Autodesk Inventor part; units mm, degrees
ref_plane "YZ Plane" through (0, 0, 0) normal (1, 0, 0) x (0, 1, 0)
ref_plane "XZ Plane" through (0, 0, 0) normal (0, 1, 0) x (-1, 0, 0)
ref_plane "XY Plane" through (0, 0, 0) normal (0, 0, 1) x (1, 0, 0)
sketch "Sketch1" plane through (0, 0, 0) normal (0, 0, 1) x (1, 0, 0)
  line L0 (0, 0) -> (-203.2, 0)
  line L1 (-203.2, 0) -> (-203.2, -1.6002)
  line L2 (-203.2, -1.6002) -> (0, -1.6002)
  line L3 (0, -1.6002) -> (0, 0)
  dimension "d0" = 203.2
  dimension "d1" = 1.6002
extrude "Extrusion1" add sketch "Sketch1" along normal blind 86.36
sketch "Sketch2" plane through (-203.2, 0, 0) normal (0, 1, 0) x (1, 0, 0)
  line L0 (203.2, 0) -> (0, 0)
  line L1 (203.2, -86.36) -> (0, -86.36)
  line L2 (0, 0) -> (1.6002, 0)
  line L3 (1.6002, 0) -> (1.6002, -86.36)
  line L4 (1.6002, -86.36) -> (0, -86.36)
  line L5 (0, -86.36) -> (0, 0)
  dimension "d4" = 1.6002
extrude "Extrusion2" add sketch "Sketch2" along normal blind 15.24
sketch "Sketch3" plane through (0, 0, 86.36) normal (0, 1, 0) x (1, 0, 0)
  line L0 (-203.2, 0) -> (0, 0)
  line L1 (-203.2, 86.36) -> (0, 86.36)
  line L2 (-150.7998, 0) -> (-149.1996, 0)
  line L3 (-149.1996, 0) -> (-149.1996, 86.36)
  line L4 (-149.1996, 86.36) -> (-150.7998, 86.36)
  line L5 (-150.7998, 86.36) -> (-150.7998, 0)
  dimension "d7" = 1.6002
extrude "Extrusion3" add sketch "Sketch3" along normal blind 15.24
sketch "Sketch4" plane through (0, 0, 86.36) normal (0, 1, 0) x (1, 0, 0)
  line L0 (-203.2, 0) -> (0, 0)
  line L1 (-203.2, 86.36) -> (0, 86.36)
  line L2 (-98.3996, 0) -> (-96.7994, 0)
  line L3 (-96.7994, 0) -> (-96.7994, 86.36)
  line L4 (-96.7994, 86.36) -> (-98.3996, 86.36)
  line L5 (-98.3996, 86.36) -> (-98.3996, 0)
  dimension "d10" = 1.6002
extrude "Extrusion4" add sketch "Sketch4" along normal blind 15.24
sketch "Sketch5" plane through (0, 0, 86.36) normal (0, 1, 0) x (1, 0, 0)
  line L0 (0, 0) -> (-96.7994, 0)
  line L1 (0, 86.36) -> (-96.7994, 86.36)
  line L2 (-45.9994, 0) -> (-44.3992, 0)
  line L3 (-44.3992, 0) -> (-44.3992, 86.36)
  line L4 (-44.3992, 86.36) -> (-45.9994, 86.36)
  line L5 (-45.9994, 86.36) -> (-45.9994, 0)
  dimension "d13" = 1.6002
extrude "Extrusion5" add sketch "Sketch5" along normal blind 15.24
sketch "Sketch6" plane through (-203.2, -1.6002, 0) normal (-1, 0, 0) x (0, 0, 1)
  line L0 (0, 0) -> (86.36, 0)
  line L1 (36.83, 0) -> (49.53, 0)
  line L2 (49.53, 0) -> (49.53, 80.01)
  line L3 (49.53, 80.01) -> (36.83, 80.01)
  line L4 (36.83, 80.01) -> (36.83, 0)
  point P0 (0, 1.6002)
  dimension "d16" = 12.7
  dimension "d17" = 80.01
extrude "Extrusion6" add sketch "Sketch6" along normal blind 1.6002
sketch "Sketch7" plane through (0, 0, 86.36) normal (1, 0, 0) x (0, 0, -1)
  line L0 (36.83, -1.6002) -> (0, -1.6002)
  line L1 (49.53, 78.4098) -> (49.53, -1.6002)
  line L2 (36.83, -1.6002) -> (49.53, -1.6002)
  line L3 (49.53, -1.6002) -> (49.53, 78.4098)
  line L4 (49.53, 78.4098) -> (36.83, 78.4098)
  line L5 (36.83, 78.4098) -> (36.83, -1.6002)
  point P0 (86.36, 0)
  dimension "d20" = 80.01
extrude "Extrusion7" add sketch "Sketch7" along normal blind 1.6002
sketch "Sketch8" plane through (-96.7994, 0, 86.36) normal (0, 1, 0) x (1, 0, 0)
  point P0 (96.7994, 86.36)
properties part number "ModulePlate2.0"
Can you work these out from the model? Positions are in its coordinate system, mm. A direction names the side the tool comes from. Give positions to 0.01 mm unless a question says otherwise; leave off trailing zeros. Order: outer loops, then holes, each group sorted by start corner. A loop starts at its lowest first (then second) coordinate and runs counter-clockwise, first axis right, second up. Notation, with made-up numbers: M -11,20 L 27,20 A26 cw 27,49 Z; hole C 1.5,-27.75 d3. An arc over 180 degrees is marked long. One line per item, written item: value.
Item 1: If we section it at C-C on x = -59: Write out the boundary of the cut face in (y, z), and give its area (3 significant figures).
Verdict:
outline: M -1.6,0 L 0,0 L 0,86.36 L -1.6,86.36 Z
area: 138 mm2
Item 2: If we section it at A-A on y = 49: Write out the boundary of the cut face in (x, z).
Verdict:
outline: M -204.8,36.83 L -203.2,36.83 L -203.2,49.53 L -204.8,49.53 Z; M 0,36.83 L 1.6,36.83 L 1.6,49.53 L 0,49.53 Z
Item 3: For faces 4 (the face through (-203.2, 7, 68)), 5 (the face through (-149.2, 8, 44)), 6 (the face through (-102, -1, 86.36)), which set-ups out of +Z, -Z, +X, -X, +Y, -Y let a thin tool reach every point of the face, with its end or its side?
Verdict:
face 4: +Z, -X, +Y, -Y
face 5: +Z, -Z, +Y
face 6: +Z, +X, -X, +Y, -Y
Item 4: If we section it at B-B on z = 56: Write out the boundary of the cut face in (x, y), and give its area (3 significant figures).
Verdict:
outline: M -203.2,-1.6 L 0,-1.6 L 0,0 L -44.4,0 L -44.4,15.24 L -46,15.24 L -46,0 L -96.8,0 L -96.8,15.24 L -98.4,15.24 L -98.4,0 L -149.2,0 L -149.2,15.24 L -150.8,15.24 L -150.8,0 L -201.6,0 L -201.6,15.24 L -203.2,15.24 Z
area: 423 mm2
Item 5: If we mould it in two halves opening along X, with no side actions, what happens to faces 1 (the face through (-150.8, 8, 43)), 2 (the face through (-204.8, 39, 43)), 3 (the face through (-103, -1.6, 44))? For each: pulls with the +X half, pulls with the -X half, needs draft (parallel to the pull), parting line crosses it, or undercut.
Verdict:
face 1: undercut
face 2: pulls with the -X half
face 3: needs draft
Item 6: Please list where these lines run through material, in increasing order: line 1 (X direction, y = 12.5, z = 19.5); line 2 (X direction, y = 44, z = 49); line 3 (Y direction, x = -42, z = 46.5).
Verdict:
line 1: -203.2 to -201.6, -150.8 to -149.2, -98.4 to -96.8, -46 to -44.4
line 2: -204.8 to -203.2, 0 to 1.6
line 3: -1.6 to 0
Item 7: For pin 1 (10 mm diameter, centred on x = -133, y = 8.5, fed in from -Z); pin 2 (1.8 mm diameter, centred on x = -202.5, z = 56, fed in from +Y); pin 3 (15 mm diameter, centred on x = -131, z = 54.5, fed in from +Y); pin 4 (1.3 mm diameter, centred on y = -1, z = 72.5, fed in from +X), each with a flat end and sliding along its axis, tell me the tip position at first contact or that it passes through.
Verdict:
pin 1: through
pin 2: y = 15.24
pin 3: y = 0
pin 4: x = 0
